```python
from build123d import *

# Parameters (mm, degrees)
BOSS_EXTRUDE1_DEPTH = 5
SKETCH3_W           = 30.7
SKETCH3_H           = 30.8
SKETCH3_W_2         = 30.3
SKETCH3_H_2         = 30.4
CUT_EXTRUDE1_DEPTH  = 10
LPATTERN1_COUNT     = 5
LPATTERN1_PITCH     = 65
SKETCH4_W           = 12
SKETCH4_H           = 5
CUT_EXTRUDE2_DEPTH  = 10
LPATTERN2_COUNT     = 5
LPATTERN2_PITCH     = 65
SKETCH5_R           = 4
CUT_EXTRUDE3_DEPTH  = 5


with BuildPart() as part:
    # Sketch1 → Boss-Extrude1 (new body)
    with BuildSketch(Plane(origin=(0, 0, 0), x_dir=(1, 0, 0), z_dir=(0, 1, 0))):
        with BuildLine():
            Line((-75, 200), (75, 200))
            ThreePointArc((75, 200), (110.355339059, 185.355339059), (125, 150))
            Line((125, 150), (125, -150))
            ThreePointArc((125, -150), (110.355339059, -185.355339059), (75, -200))
            Line((75, -200), (-75, -200))
            ThreePointArc((-75, -200), (-110.355339059, -185.355339059), (-125, -150))
            Line((-125, -150), (-125, 150))
            ThreePointArc((-125, 150), (-110.355339059, 185.355339059), (-75, 200))
        make_face()
    extrude(amount=BOSS_EXTRUDE1_DEPTH)

    # Sketch3 → Cut-Extrude1 (cut)
    # profile 1 of 4: a face of its own
    with BuildSketch(Plane.XZ):
        with Locations((-75.225, 129.928570167)):
            Rectangle(SKETCH3_W, SKETCH3_H)
        with Locations((-75.225, 129.928570167)):
            Rectangle(SKETCH3_W_2, SKETCH3_H_2, mode=Mode.SUBTRACT)
    # profile 2 of 4: a face of its own
    with BuildSketch(Plane.XZ):
        with Locations((-75.225, 129.928570167)):
            Rectangle(SKETCH3_W_2, SKETCH3_H_2)
    # profile 3 of 4: a face of its own
    with BuildSketch(Plane.XZ):
        with Locations((75.225, 129.928570167)):
            Rectangle(SKETCH3_W, SKETCH3_H)
        with Locations((75.225, 129.928570167)):
            Rectangle(SKETCH3_W_2, SKETCH3_H_2, mode=Mode.SUBTRACT)
    # profile 4 of 4: a face of its own
    with BuildSketch(Plane.XZ):
        with Locations((75.225, 129.928570167)):
            Rectangle(SKETCH3_W_2, SKETCH3_H_2)
    cut_extrude1 = extrude(amount=-CUT_EXTRUDE1_DEPTH, mode=Mode.SUBTRACT)

    # LPattern1: Cut-Extrude1 ×5
    with Locations(*[(0, 0, -i * LPATTERN1_PITCH) for i in range(1, LPATTERN1_COUNT)]):
        add(cut_extrude1, mode=Mode.SUBTRACT)

    # Sketch4 → Cut-Extrude2 (cut)
    with BuildSketch(Plane(origin=(0, 5, 0), x_dir=(1, 0, 0), z_dir=(0, 1, 0))):
        with Locations((-48.165, -139.42)):
            Rectangle(SKETCH4_W, SKETCH4_H)
        with Locations((-48.165, -121.42)):
            Rectangle(SKETCH4_W, SKETCH4_H)
        with Locations((48.165, -139.42)):
            Rectangle(SKETCH4_W, SKETCH4_H)
        with Locations((48.165, -121.42)):
            Rectangle(SKETCH4_W, SKETCH4_H)
    cut_extrude2 = extrude(amount=-CUT_EXTRUDE2_DEPTH, mode=Mode.SUBTRACT)

    # LPattern2: Cut-Extrude2 ×5
    with Locations(*[(0, 0, -i * LPATTERN2_PITCH) for i in range(1, LPATTERN2_COUNT)]):
        add(cut_extrude2, mode=Mode.SUBTRACT)

    # Sketch5 → Cut-Extrude3 (cut)
    with BuildSketch(Plane(origin=(0, 5, 0), x_dir=(1, 0, 0), z_dir=(0, 1, 0))):
        with Locations(Location((-103, 170, 0), (0, 0, 270))):
            Circle(SKETCH5_R)
        with Locations(Location((103, 170, 0), (0, 0, 270))):
            Circle(SKETCH5_R)
        with Locations(Location((103, -170, 0), (0, 0, 270))):
            Circle(SKETCH5_R)
        with Locations(Location((-103, -170, 0), (0, 0, 270))):
            Circle(SKETCH5_R)
        with Locations(Location((-112, 0, 0), (0, 0, 270))):
            Circle(SKETCH5_R)
        with Locations(Location((112, 0, 0), (0, 0, 270))):
            Circle(SKETCH5_R)
    extrude(amount=-CUT_EXTRUDE3_DEPTH, mode=Mode.SUBTRACT)


solid = part.part
```
Input: part model. Units: mm. Frame: model coordinates. Give positions to 0.01 mm unless a question says otherwise; leave off trailing zeros. Order: outer loops, then holes, each group sorted by start corner. A loop starts at its lowest first (then second) coordinate and runs counter-clockwise, first axis right, second up. Notation, with made-up numbers: (-2, -30.75) - (29, -30.75) arc R20 ccw to (29, -2.75) - close; hole circle Ø6 at (78.25, -39.5). An arc over 180 degrees is marked (long way). Use a Markdown table: item, result.
(1) Section query C-C (y = 1.35). State how many separate pieces and enclosed holes the cut face has, then the cut area to 3 significant figures.
Computed values:
| item | result |
|---|---|
| separate pieces | 1 |
| enclosed holes | 36 |
| area | 86,900 mm2 |
(2) Section query D-D (x = -103). Output: boundary loops of the cut face in (y, z).
Computed values:
| item | result |
|---|---|
| outline | (0, -191.42) - (5, -191.42) - (5, -174) - (0, -174) - close; (0, -166) - (5, -166) - (5, 166) - (0, 166) - close; (0, 174) - (5, 174) - (5, 191.42) - (0, 191.42) - close |
(3) Section query B-B (x = 112). Output: boundary loops of the cut face in (y, z), then the cut area to 3 significant figures.
Computed values:
| item | result |
|---|---|
| outline | (0, -183.63) - (5, -183.63) - (5, -4) - (0, -4) - close; (0, 4) - (5, 4) - (5, 183.63) - (0, 183.63) - close |
| area | 1,800 mm2 |
(4) Draft query along X for faces 1 (the cylindrical face through (101.468, 2.535, -166.305)), 2 (the cylindrical face through (-110.742, 2.465, -184.964)), 3 (the flat face through (2, 0, -3)). Return one class per face: released by +X, released by -X, zero draft, split by the parting line, or undercut.
Computed values:
| item | result |
|---|---|
| face 1 | undercut |
| face 2 | released by -X |
| face 3 | zero draft |
(5) Line query: line 1 (Z direction, x = 64.5, y = 1.5); line 2 (X direction, y = 3.1, z = 0) (3 decimals); line 3 (X direction, y = 3.75, z = -73) (3 decimals). Output: solid intervals per line, ascending. Write a range as from..to.
Computed values:
| item | result |
|---|---|
| line 1 | z = -200..-145.47, -114.67..-80.47, -49.67..-15.47, 15.33..49.53, 80.33..114.53, 145.33..200 |
| line 2 | x = -125..-116, -108..-90.575, -59.875..59.875, 90.575..108, 116..125 |
| line 3 | x = -125..-90.575, -59.875..-54.165, -42.165..42.165, 54.165..59.875, 90.575..125 |
(6) Section query A-A (z = 0). Output: boundary loops of the cut face in (x, y) (3 decimals), then the cut area to 3 significant figures.
Computed values:
| item | result |
|---|---|
| outline | (-125, 0) - (-116, 0) - (-116, 5) - (-125, 5) - close; (-108, 0) - (-90.575, 0) - (-90.575, 5) - (-108, 5) - close; (-59.875, 0) - (59.875, 0) - (59.875, 5) - (-59.875, 5) - close; (90.575, 0) - (108, 0) - (108, 5) - (90.575, 5) - close; (116, 0) - (125, 0) - (125, 5) - (116, 5) - close |
| area | 863 mm2 |
(7) Pin query (flat end, axial travel): pin 1 (2 mm diameter, centred on y = 4, z = 152.5, fed in from +X). Return the tip coordinate at first contact, or that it passes through.
Computed values:
| item | result |
|---|---|
| pin 1 | stops at x = 124.98 |
